Model file for the job. Use its own axes, mm. A direction names the side the tool comes from. Round coordinates to 2 decimals unless told otherwise and drop trailing zeros. Loops run counter-clockwise (first coordinate to the right, second up) from the corner with the lowest first, then second, coordinate; pieces in that order, holes last. Notation, with made-up numbers: (64.5, 89) -> (102.5, 89) arc R26 ccw to (102.5, 127) -> close; hole circle Ø1 at (4, 50.25). An arc over 180 degrees is marked (long way). Use a Markdown table: item, result. Add a question column.
```python
from build123d import *

# Parameters (mm, degrees)
SKETCH1_W           = 75
SKETCH1_H           = 35
MAINSHAPE_DEPTH     = 4.5
SKETCH2_W           = 4.5
SKETCH2_H           = 10
REARTAB_DEPTH       = 4.5
SKETCH3_W           = 10
SKETCH3_H           = 4.5
BOSS_EXTRUDE3_DEPTH = 4.5
CUT_EXTRUDE1_DEPTH  = 83.886971232
SKETCH6_R           = 14
SKETCH6_R_2         = 1.55
CUT_EXTRUDE3_DEPTH  = 83.886971232
BOSS_EXTRUDE4_DEPTH = 4.5
CUT_EXTRUDE7_DEPTH  = 85.433901689
SMOOTHEDGE_DEPTH    = 85.433901689


with BuildPart() as part:
    # Sketch1 → MainShape (new body)
    with BuildSketch(Plane.XY):
        with Locations((37.5, -17.5)):
            Rectangle(SKETCH1_W, SKETCH1_H)
    extrude(amount=MAINSHAPE_DEPTH)

    # Sketch2 → RearTab (add, through all)
    with BuildSketch(Plane.XY.offset(4.5)):
        with Locations((-2.25, -7.5)):
            Rectangle(SKETCH2_W, SKETCH2_H)
    extrude(amount=-REARTAB_DEPTH)

    # Sketch3 → Boss-Extrude3 (add, through all)
    with BuildSketch(Plane.XY.offset(4.5)):
        with Locations((15, 2.25)):
            Rectangle(SKETCH3_W, SKETCH3_H)
        with Locations((55, 2.25)):
            Rectangle(SKETCH3_W, SKETCH3_H)
    extrude(amount=-BOSS_EXTRUDE3_DEPTH)

    # Sketch4 → Cut-Extrude1 (cut, through all)
    with BuildSketch(Plane.XY.offset(4.5)):
        with BuildLine():
            Line((67.25, 0), (67.25, -3.8))
            Line((67.25, -3.8), (66.25, -3.8))
            ThreePointArc((66.25, -3.8), (66.073223305, -3.873223305), (66, -4.05))
            Line((66, -4.05), (66, -7.75))
            ThreePointArc((66, -7.75), (66.073223305, -7.926776695), (66.25, -8))
            Line((66.25, -8), (67.25, -8))
            Line((67.25, -8), (67.25, -10.5))
            Line((67.25, -10.5), (70.75, -10.5))
            Line((70.75, -10.5), (70.75, -8))
            Line((70.75, -8), (71.75, -8))
            ThreePointArc((71.75, -8), (71.926776695, -7.926776695), (72, -7.75))
            Line((72, -7.75), (72, -4.05))
            ThreePointArc((72, -4.05), (71.926776695, -3.873223305), (71.75, -3.8))
            Line((71.75, -3.8), (70.75, -3.8))
            Line((70.75, -3.8), (70.75, 0))
            Line((70.75, 0), (67.25, 0))
        make_face()
    extrude(amount=-CUT_EXTRUDE1_DEPTH, mode=Mode.SUBTRACT)

    # Sketch6 → Cut-Extrude3 (cut, through all)
    with BuildSketch(Plane.XY.offset(4.5)):
        with Locations((52, -20)):
            Circle(SKETCH6_R)
        with Locations((40, -8)):
            Circle(SKETCH6_R_2)
        with Locations((64, -32)):
            Circle(SKETCH6_R_2)
        with Locations((40, -32)):
            Circle(SKETCH6_R_2)
    extrude(amount=-CUT_EXTRUDE3_DEPTH, mode=Mode.SUBTRACT)

    # Sketch7 → Boss-Extrude4 (add, through all)
    with BuildSketch(Plane.XY.offset(4.5)):
        with BuildLine():
            Line((62.86329805, -35), (41.13670195, -35))
            ThreePointArc((41.13670195, -35), (52, -38.520562748), (62.86329805, -35))
        make_face()
    extrude(amount=-BOSS_EXTRUDE4_DEPTH)

    # Sketch11 → Cut-Extrude7 (cut, through all)
    with BuildSketch(Plane.XY.offset(4.5)):
        with BuildLine():
            Line((0, -31.25), (0, -27.75))
            Line((0, -27.75), (3.8, -27.75))
            Line((3.8, -27.75), (3.8, -26.75))
            ThreePointArc((3.8, -26.75), (3.873223305, -26.573223305), (4.05, -26.5))
            Line((4.05, -26.5), (7.75, -26.5))
            ThreePointArc((7.75, -26.5), (7.926776695, -26.573223305), (8, -26.75))
            Line((8, -26.75), (8, -27.75))
            Line((8, -27.75), (10.5, -27.75))
            Line((10.5, -27.75), (10.5, -31.25))
            Line((10.5, -31.25), (8, -31.25))
            Line((8, -31.25), (8, -32.25))
            ThreePointArc((8, -32.25), (7.926776695, -32.426776695), (7.75, -32.5))
            Line((7.75, -32.5), (4.05, -32.5))
            ThreePointArc((4.05, -32.5), (3.873223305, -32.426776695), (3.8, -32.25))
            Line((3.8, -32.25), (3.8, -31.25))
            Line((3.8, -31.25), (0, -31.25))
        make_face()
    extrude(amount=-CUT_EXTRUDE7_DEPTH, mode=Mode.SUBTRACT)

    # Sketch14 → SmoothEdge (cut, through all)
    with BuildSketch(Plane.XY.offset(4.5)):
        with BuildLine():
            Line((69.435595774, -35), (75, -35))
            Line((75, -35), (75, -20))
            ThreePointArc((75, -20), (73.564075482, -27.999415516), (69.435595774, -35))
        make_face()
    extrude(amount=-SMOOTHEDGE_DEPTH, mode=Mode.SUBTRACT)


solid = part.part
```
1) Cut at A-A on x = 52. Write the cut outline in (y, z).
2) Pull direction Y, two halves, no side cores. Call faces 5 (the face through (73, 0, 2)), 6 (the face through (66, -35, 2)), 7 (the face through (0, -20, 2)), 8 (the face through (40.83, -30.69, 2.28)): +Y half, -Y half, draft (parallel to the pull), parting line (faces both ways), or undercut.
3) Tool access for faces 1 (the face through (67.25, -2, 2)), 2 (the face through (10.5, -29, 2)), 3 (the face through (0, -33, 2)), 4 (the face through (6, -26.5, 2)): list every direction of +Z, -Z, +X, -X, +Y, -Y with a clear straight run to the whole face (end or side of a thin tool).
4) Cut at D-D on z = 3.4. Count the separate pieces of the cut face and the enclosed holes in it, and give its area (3 significant figures).
5) Cut at B-B on x = 64. Write the cut outline in (y, z), and give its area (4 significant figures).
6) Pin check, flat tips, straight feed: pin 1 Ø1.1 at (y, z) = (-33, 2) entering from -X; pin 2 Ø2 at (x, z) = (72, 2.5) entering from +Y; pin 3 Ø1.1 at (y, z) = (-27.5, 1.5) entering from +X; pin 4 Ø3 at (x, y) = (40, -8) entering from -Z. Stop position of each tip, or through.
7) Cut at C-C on x = 40. Write the cut outline in (y, z), and give its area (3 significant figures).
8) Wall check: probe 1 along Y at (x, z) = (52, 2); probe 2 along X at (y, z) = (2, 4.2); probe 3 along Y at (x, z) = (9, 1.5). Give the ranges that are in metal, low to high. Write a range as from..to.
Established:
| question | item | result |
|---|---|---|
| 1 | outline | (-38.52, 0) -> (-34, 0) -> (-34, 4.5) -> (-38.52, 4.5) -> close; (-6, 0) -> (4.5, 0) -> (4.5, 4.5) -> (-6, 4.5) -> close |
| 2 | face 5 | +Y half |
| 2 | face 6 | -Y half |
| 2 | face 7 | draft |
| 2 | face 8 | undercut |
| 3 | face 1 | +Z, -Z, +Y |
| 3 | face 2 | +Z, -Z, -X |
| 3 | face 3 | +Z, -Z, -X, -Y |
| 3 | face 4 | +Z, -Z |
| 4 | separate pieces | 1 |
| 4 | enclosed holes | 4 |
| 4 | area | 2,050 mm^2 |
| 5 | outline | (-35, 0) -> (-33.55, 0) -> (-33.55, 4.5) -> (-35, 4.5) -> close; (-30.45, 0) -> (-27.21, 0) -> (-27.21, 4.5) -> (-30.45, 4.5) -> close; (-12.79, 0) -> (0, 0) -> (0, 4.5) -> (-12.79, 4.5) -> close |
| 5 | area | 78.65 mm^2 |
| 6 | pin 1 | stops at x = 0 |
| 6 | pin 2 | stops at y = 0 |
| 6 | pin 3 | stops at x = 73.92 |
| 6 | pin 4 | passes through |
| 7 | outline | (-35, 0) -> (-33.55, 0) -> (-33.55, 4.5) -> (-35, 4.5) -> close; (-30.45, 0) -> (-27.21, 0) -> (-27.21, 4.5) -> (-30.45, 4.5) -> close; (-12.79, 0) -> (-9.55, 0) -> (-9.55, 4.5) -> (-12.79, 4.5) -> close; (-6.45, 0) -> (0, 0) -> (0, 4.5) -> (-6.45, 4.5) -> close |
| 7 | area | 64.7 mm^2 |
| 8 | probe 1 | y = -38.52..-34, -6..4.5 |
| 8 | probe 2 | x = 10..20, 50..60 |
| 8 | probe 3 | y = -35..-31.25, -27.75..0 |
